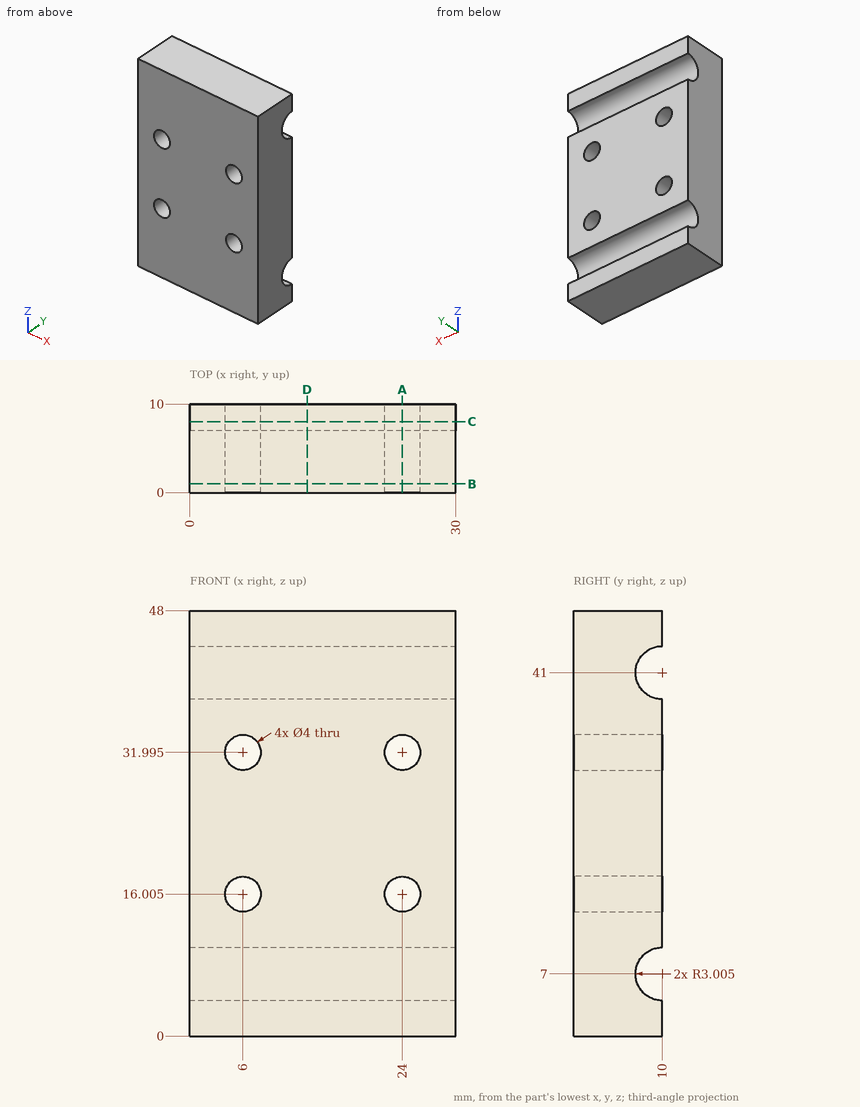
Here's the drawing with two shaded views (mm, measured from the low corner). I have some questions. Give positions to 0.01 mm unless a question says otherwise; leave off trailing zeros. Order: outer loops, then holes, each group sorted by start corner. A loop starts at its lowest first (then second) coordinate and runs counter-clockwise, first axis right, second up. Notation, with made-up numbers: (67.5, -25) -> (97.5, -25) arc R25 cw to (97.5, 10) -> close; hole circle Ø3 at (85.25, 11.25). An arc over 180 degrees is marked (long way). Use a Markdown table: item, result. Add a question column.
Item 1: Imagine slicing it at A-A on x = 24. Please give me the cut outline in (y, z) (3 decimals).
Item 2: Will this pin go through, and if not, where does the flat tip stop? pin 1 (2.5 mm diameter, centred on x = 24, z = 31.995, fed in from -Y).
Item 3: Imagine slicing it at C-C on y = 8. Please give me the cut outline in (x, z) (3 decimals).
Item 4: I need wall thicknesses on line 1 (X direction, y = 2, z = 14.5); line 2 (Z direction, x = 22.75, y = 8); line 3 (Z direction, x = 2.25, y = 8.5). Which ranges of each line are inside material? Lowest first, please.
Item 5: Imagine slicing it at B-B on y = 1. Please give me the cut outline in (x, z) (3 decimals).
Item 6: Imagine slicing it at D-D on x = 13.25. Please give me the cut outline in (y, z) (3 decimals), plus the area to 3 significant figures.
Data:
| question | item | result |
|---|---|---|
| 1 | outline | (0, 0) -> (10, 0) -> (10, 3.995) arc R3.005 cw to (10, 10.005) -> (10, 14.005) -> (0, 14.005) -> close; (0, 18.005) -> (10, 18.005) -> (10, 29.995) -> (0, 29.995) -> close; (0, 33.995) -> (10, 33.995) -> (10, 37.995) arc R3.005 cw to (10, 44.005) -> (10, 48) -> (0, 48) -> close |
| 2 | pin 1 | passes through |
| 3 | outline | (0, 0) -> (30, 0) -> (30, 4.757) -> (0, 4.757) -> close; (0, 9.243) -> (30, 9.243) -> (30, 38.757) -> (0, 38.757) -> close; (0, 43.243) -> (30, 43.243) -> (30, 48) -> (0, 48) -> close; hole circle Ø4 at (6, 16.005); hole circle Ø4 at (6, 31.995); hole circle Ø4 at (24, 16.005); hole circle Ø4 at (24, 31.995) |
| 4 | line 1 | x = 0 to 4.68, 7.32 to 22.68, 25.32 to 30 |
| 4 | line 2 | z = 0 to 4.76, 9.24 to 14.44, 17.57 to 30.43, 33.56 to 38.76, 43.24 to 48 |
| 4 | line 3 | z = 0 to 4.4, 9.6 to 38.4, 43.6 to 48 |
| 5 | outline | (0, 0) -> (30, 0) -> (30, 48) -> (0, 48) -> close; hole circle Ø4 at (6, 16.005); hole circle Ø4 at (6, 31.995); hole circle Ø4 at (24, 16.005); hole circle Ø4 at (24, 31.995) |
| 6 | outline | (0, 0) -> (10, 0) -> (10, 3.995) arc R3.005 cw to (10, 10.005) -> (10, 37.995) arc R3.005 cw to (10, 44.005) -> (10, 48) -> (0, 48) -> close |
| 6 | area | 452 mm² |
